For this review, take the finished solid that the model builds, in its own axes (mm). Face numbers are marked on the shaded views. A direction names the side the tool comes from. Round coordinates to 2 decimals unless told otherwise and drop trailing zeros. Order: outer loops, then holes, each group sorted by start corner. A loop starts at its lowest first (then second) coordinate and runs counter-clockwise, first axis right, second up. Notation, with made-up numbers: (87, 70) - (105, 70) arc R32 ccw to (105, 100) - close; hole circle Ø7 at (-35, -12). An arc over 180 degrees is marked (long way). One line per question, with ' | ' between items.
```python
from build123d import *

# Parameters (mm, degrees)
SKETCH2_W           = 71.4
SKETCH2_H           = 93
SKETCH2_W_2         = 51.4
SKETCH2_H_2         = 73
BOSS_EXTRUDE1_DEPTH = 10
SKETCH3_W           = 14
SKETCH3_H           = 26
SKETCH3_R           = 2.75
BOSS_EXTRUDE2_DEPTH = 5
SKETCH4_R           = 3.95
SKETCH4_R_2         = 2.75
BOSS_EXTRUDE3_DEPTH = 8.4
SKETCH5_W           = 51.4
SKETCH5_H           = 10
CUT_EXTRUDE1_DEPTH  = 65.130647899
SKETCH6_R           = 5.15
SKETCH6_R_2         = 3.95
BOSS_EXTRUDE4_DEPTH = 0.4
SKETCH7_W           = 71.4
SKETCH7_H           = 25
CUT_EXTRUDE2_DEPTH  = 65.130647899
FILLET1_START       = -46.5
FILLET1_DEPTH       = 5
FILLET1_2_DEPTH     = 5
SKETCH10_W          = 71.4
SKETCH10_H          = 58
CUT_EXTRUDE3_DEPTH  = 65.130647899
SKETCH9_R           = 2.55
CUT_EXTRUDE4_DEPTH  = 53.440919138
FILLET2_R           = 5
SKETCH11_R          = 2.75
BOSS_EXTRUDE5_DEPTH = 13.4
CHAMFER1_SIZE       = 0.5


with BuildPart() as part:
    # Sketch2 → Boss-Extrude1 (new body)
    with BuildSketch(Plane(origin=(0, 0, 0), x_dir=(1, 0, 0), z_dir=(0, 1, 0))):
        Rectangle(SKETCH2_W, SKETCH2_H)
        Rectangle(SKETCH2_W_2, SKETCH2_H_2, mode=Mode.SUBTRACT)
    extrude(amount=BOSS_EXTRUDE1_DEPTH)

    # Sketch3 → Boss-Extrude2 (add)
    with BuildSketch(Plane(origin=(0, 0, -46.5), x_dir=(-1, 0, 0), z_dir=(0, 0, -1))):
        with Locations((0, 23)):
            Rectangle(SKETCH3_W, SKETCH3_H)
        with Locations((0, 30)):
            Circle(SKETCH3_R, mode=Mode.SUBTRACT)
    extrude(amount=-BOSS_EXTRUDE2_DEPTH)

    # Sketch4 → Boss-Extrude3 (add)
    with BuildSketch(Plane.XY.offset(-41.5)):
        with Locations(Location((0, 30, 0), (0, 0, 180))):
            Circle(SKETCH4_R)
        with Locations(Location((0, 30, 0), (0, 0, 180))):
            Circle(SKETCH4_R_2, mode=Mode.SUBTRACT)
    extrude(amount=BOSS_EXTRUDE3_DEPTH)

    # Sketch5 → Cut-Extrude1 (cut, through all)
    with BuildSketch(Plane(origin=(0, 10, 0), x_dir=(1, 0, 0), z_dir=(0, 1, 0))):
        with Locations((0, -41.5)):
            Rectangle(SKETCH5_W, SKETCH5_H)
    extrude(amount=-CUT_EXTRUDE1_DEPTH, mode=Mode.SUBTRACT)

    # Sketch6 → Boss-Extrude4 (add)
    with BuildSketch(Plane.XY.offset(-41.5)):
        with Locations(Location((0, 30, 0), (0, 0, 180))):
            Circle(SKETCH6_R)
        with Locations((0, 30)):
            Circle(SKETCH6_R_2, mode=Mode.SUBTRACT)
    extrude(amount=BOSS_EXTRUDE4_DEPTH)

    # Sketch7 → Cut-Extrude2 (cut, through all)
    with BuildSketch(Plane(origin=(0, 10, 0), x_dir=(1, 0, 0), z_dir=(0, 1, 0))):
        with Locations((0, -34)):
            Rectangle(SKETCH7_W, SKETCH7_H)
    extrude(amount=-CUT_EXTRUDE2_DEPTH, mode=Mode.SUBTRACT)

    # Fillet1: read off the stored shape, not the designer's step
    # Fillet1 outline → Fillet1 (cut)
    with BuildSketch(Plane.XY.offset(FILLET1_START)):
        with BuildLine():
            ThreePointArc((0, 36), (4.949747468, 33.949747468), (7, 29))
            Line((7, 29), (7, 36))
            Line((7, 36), (0, 36))
        make_face()
        with BuildLine():
            ThreePointArc((-7, 29), (-4.949747468, 33.949747468), (0, 36))
            Line((0, 36), (-7, 36))
            Line((-7, 36), (-7, 29))
        make_face()
    extrude(amount=FILLET1_DEPTH, mode=Mode.SUBTRACT)

    # Fillet1 2 outline → Fillet1 2 (add)
    with BuildSketch(Plane.XY.offset(FILLET1_START)):
        with BuildLine():
            ThreePointArc((14, 10), (9.050252532, 12.050252532), (7, 17))
            Line((7, 17), (7, 10))
            Line((7, 10), (14, 10))
        make_face()
        with BuildLine():
            Line((-14, 10), (-7, 10))
            Line((-7, 10), (-7, 17))
            ThreePointArc((-7, 17), (-9.050252532, 12.050252532), (-14, 10))
        make_face()
    extrude(amount=FILLET1_2_DEPTH)

    # Sketch10 → Cut-Extrude3 (cut, through all)
    with BuildSketch(Plane(origin=(0, 10, 0), x_dir=(1, 0, 0), z_dir=(0, 1, 0))):
        with Locations((0, 7.5)):
            Rectangle(SKETCH10_W, SKETCH10_H)
    extrude(amount=-CUT_EXTRUDE3_DEPTH, mode=Mode.SUBTRACT)

    # Sketch9 → Cut-Extrude4 (cut, through all)
    with BuildSketch(Plane(origin=(0, 0, -46.5), x_dir=(-1, 0, 0), z_dir=(0, 0, -1))):
        with Locations((-28.2, 5)):
            Circle(SKETCH9_R)
        with Locations((28.2, 5)):
            Circle(SKETCH9_R)
    extrude(amount=-CUT_EXTRUDE4_DEPTH, mode=Mode.SUBTRACT)

    # Fillet2
    fillet2_edges = [part.edges().sort_by_distance(p)[0] for p in [
        (-35.7, 10, -41.5),
        (-35.7, 0, -41.5),
        (35.7, 0, -41.5),
        (35.7, 10, -41.5),
    ]]
    fillet(fillet2_edges, radius=FILLET2_R - 0.0001)  # a hair under: the kernel refuses the full size

    # Sketch11 → Boss-Extrude5 (add)
    with BuildSketch(Plane(origin=(0, 0, -46.5), x_dir=(-1, 0, 0), z_dir=(0, 0, -1))):
        with Locations((0, 30)):
            Circle(SKETCH11_R)
        with BuildLine():
            Line((-2.05, 31.516575089), (-2.05, 28.483424911))
            ThreePointArc((-2.05, 28.483424911), (0, 27.45), (2.05, 28.483424911))
            Line((2.05, 28.483424911), (2.05, 31.516575089))
            ThreePointArc((2.05, 31.516575089), (0, 32.55), (-2.05, 31.516575089))
        make_face(mode=Mode.SUBTRACT)
    extrude(amount=-BOSS_EXTRUDE5_DEPTH)

    # Chamfer1
    chamfer1_edges = [part.edges().sort_by_distance(p)[0] for p in [
        (0, 32.55, -46.5),
        (-2.05, 30, -46.5),
        (0, 27.45, -46.5),
        (2.05, 30, -46.5),
    ]]
    chamfer(chamfer1_edges, length=CHAMFER1_SIZE)


solid = part.part
```
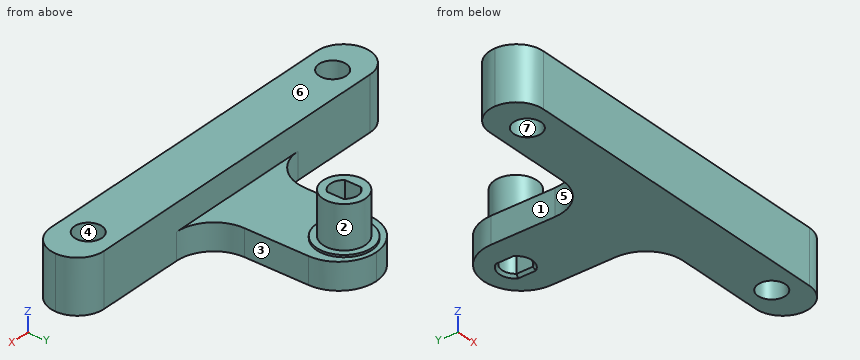
(1) We need section B-B on x = -28.2. State the section outline as (y, z) points.
Output values:
outline: (0, -46.5) - (2.45, -46.5) - (2.45, -36.5) - (0, -36.5) - close; (7.55, -46.5) - (10, -46.5) - (10, -36.5) - (7.55, -36.5) - close
(2) For probe 1 along Y at (x, z) = (-28.2, -41.75); probe 2 along X at (y, z) = (17, -45.25); probe 3 along Y at (x, z) = (14.5, -45.75), list the stretches that pass through material, from the lowest coordinate up. Write a range as [from, to].
Output values:
probe 1: [0, 2.45], [7.55, 10] | probe 2: [-7, 7] | probe 3: [0, 10]
(3) Mouldability with a two-part tool opening along X and no side actions: class the marked faces 5, 6 and 7 as released by +X, released by -X, zero draft, split by the parting line, or undercut.
Output values:
face 5: released by -X | face 6: zero draft | face 7: undercut
(4) We need section A-A on z = -39.25. Give the number of separate pieces and of enclosed holes in the cut face, plus the area to 3 significant figures.
Output values:
separate pieces: 2 | enclosed holes: 3 | area: 682 mm^2
(5) We need section D-D on y = 30. State the section outline as (x, z) points, plus the area to 3 significant figures.
Output values:
outline: (-6.93, -46.5) - (-2.55, -46.5) - (-2.05, -46) - (-2.05, -33.1) - (-3.95, -33.1) - (-3.95, -41.1) - (-5.15, -41.1) - (-5.15, -41.5) - (-6.93, -41.5) - close; (2.05, -46) - (2.55, -46.5) - (6.93, -46.5) - (6.93, -41.5) - (5.15, -41.5) - (5.15, -41.1) - (3.95, -41.1) - (3.95, -33.1) - (2.05, -33.1) - close | area: 81.4 mm^2
(6) Insertion check: pin 1 (0.9 mm diameter, centred on y = 29.5, z = -41, fed in from -X); pin 2 (1.5 mm diameter, centred on y = 29.5, z = -39, fed in from +X); pin 3 (3 mm diameter, centred on x = -17, y = 3.5, fed in from +Z). Each pin has a flat end and moves straight along its axis. Give the tip position at first contact, or say it passes through.
Output values:
pin 1: x = -5.15 | pin 2: x = 3.95 | pin 3: z = -36.5
(7) We need section C-C on z = -35.25. State the section outline as (x, y) points, plus the area to 3 significant figures.
Output values:
outline: circle Ø7.9 at (0, 30); hole (-2.05, 28.48) arc R2.55 ccw to (2.05, 28.48) - (2.05, 31.52) arc R2.55 ccw to (-2.05, 31.52) - close | area: 30.7 mm^2
(8) For the marked faces 1, 2, 3 and 4, list the 3-axis set-ups (+Z, -Z, +X, -X, +Y, -Y) from which the entire face can be reached by the end or side of a thin tool; tool diameter is ignored.
Output values:
face 1: +Z, -Z, -X, +Y | face 2: +Z | face 3: +Z, -Z, +X, +Y | face 4: +Z, -Z
